Geometry check sheet. Reference: the model listing, model coordinates, mm. A direction names the side the tool comes from. Round coordinates to 2 decimals unless told otherwise and drop trailing zeros. Write each loop counter-clockwise with the first axis right and the second up, starting at its lowest first coordinate (ties: lowest second). Pieces come first, ordered by that corner, then holes.
Item 1: Cross-section at B-B (z = 44). Enter the section's corners in (x, y) (3 decimals), then the cut area to 3 significant figures.
Item 2: Cross-section at D-D (x = -25.5). Enter the section's corners in (y, z) (3 decimals).
Item 3: Access from +Z, -Z, +X, -X, +Y, -Y to the whole of each face (thin tool, end or side, straight path). Record for faces 1 (the face through (39.792, 7, 25)), 2 (the face through (66.286, -27.049, 10.43)), 3 (the face through (6, -10.997, 42)), 4 (the face through (-45.794, -30, 23)), 5 (the face through (-26.883, 7, 25)).
Item 4: Scan lines: probe 1 along X at (y, z) = (-36, 23); probe 2 along X at (y, z) = (-37, 5.5); probe 3 along Z at (x, y) = (-30.5, 4) (3 decimals). Record each from-to range of solid material in increasing order.
Item 5: Draft check along X on faces 6 (the face through (-54.41, -11.95, 30.41)), 7 (the face through (4, -20.522, 23)), 8 (the face through (4, -8, 0)). Enter one of: pulls with the +X half, pulls with the -X half, needs draft (parallel to the pull), parting line crosses it, or undercut.
Item 6: Cross-section at A-A (y = -22). Enter the section's corners in (x, z) (3 decimals).
Item 7: Cross-section at C-C (y = -5). Enter the section's corners in (x, z) (3 decimals).
Item 8: Depth check by flat-ended pin: P1, Ø20.5, axis at y = -24.5, z = 33.5, coming from the -X side; P2, Ø2, axis at x = 14, z = 34, coming from the -Y side; P3, Ø16.5, axis at x = 7, y = 6.5, coming from the +Z side; P4, Ø8.5, axis at x = 62.16, y = 9.35, coming from the -Z side. Enter the tip coordinate at first touch or a pass-through.
from build123d import *

# Parameters (mm, degrees)
SKETCH1_R             = 7.14375
BOSS_EXTRUDE1_DEPTH   = 9.525
BOSS_EXTRUDE1_2_DEPTH = 9.525
BOSS_EXTRUDE2_DEPTH   = 47.625
BOSS_EXTRUDE3_DEPTH   = 38.1
FILLET1_R             = 3.175


with BuildPart() as part:
    # Sketch1 → Boss-Extrude1 (new body)
    with BuildSketch(Plane.XY):
        Polygon((-26.883211679, -10.996624088), (-26.883211679, 22.340875912), (-71.194160584, 22.340875912), (-71.194160584, -39.571624088), (-55.319160584, -39.571624088), (-55.319160584, -10.996624088), align=None)
        with Locations(Location((-52.144160584, 8.053375912, 0), (0, 0, 180))):
            Circle(SKETCH1_R, mode=Mode.SUBTRACT)
    extrude(amount=BOSS_EXTRUDE1_DEPTH)



with BuildPart() as body_2:
    # Sketch1 → Boss-Extrude1 2 (new body)
    with BuildSketch(Plane.XY):
        Polygon((39.791788321, 22.340875912), (39.791788321, -10.996624088), (65.330839416, -10.996624088), (65.330839416, -39.571624088), (81.205839416, -39.571624088), (81.205839416, 22.340875912), align=None)
        with Locations(Location((62.155839416, 9.351186131, 0), (0, 0, 180))):
            Circle(SKETCH1_R, mode=Mode.SUBTRACT)
    extrude(amount=BOSS_EXTRUDE1_2_DEPTH)


with BuildPart() as part_1:
    add(part.part)

    add(body_2.part)  # Boss-Extrude2 merges body 2
    # Sketch1_4 → Boss-Extrude2 (add)
    with BuildSketch(Plane.XY):
        Polygon((39.791788321, -10.996624088), (-26.883211679, -10.996624088), (-55.319160584, -10.996624088), (-55.319160584, -39.571624088), (-45.794160584, -39.571624088), (-45.794160584, -37.984124088), (-45.794160584, -20.521624088), (55.805839416, -20.521624088), (55.805839416, -37.984124088), (55.805839416, -39.571624088), (65.330839416, -39.571624088), (65.330839416, -10.996624088), align=None)
    extrude(amount=BOSS_EXTRUDE2_DEPTH)

    # Sketch1_5 → Boss-Extrude3 (add)
    with BuildSketch(Plane.XY):
        with BuildLine():
            Line((-17.219160584, 22.340875912), (-26.883211679, 22.340875912))
            Line((-26.883211679, 22.340875912), (-26.883211679, -10.996624088))
            Line((-26.883211679, -10.996624088), (39.791788321, -10.996624088))
            Line((39.791788321, -10.996624088), (39.791788321, 22.340875912))
            Line((39.791788321, 22.340875912), (27.230839416, 22.340875912))
            ThreePointArc((27.230839416, 22.340875912), (5.005839416, 0.115875912), (-17.219160584, 22.340875912))
        make_face()
    extrude(amount=BOSS_EXTRUDE3_DEPTH)

    # Fillet1
    fillet1_edges = [part_1.edges().sort_by_distance(p)[0] for p in [
        (-41.101186131, -10.996624088, 9.525),
        (-26.883211679, 5.672125912, 9.525),
        (65.330839416, -10.996624088, 28.575),
        (-55.319160584, -10.996624088, 28.575),
        (39.791788321, 5.672125912, 9.525),
        (52.561313869, -10.996624088, 9.525),
        (65.330839416, -25.284124088, 9.525),
        (-26.883211679, -10.996624088, 23.8125),
        (39.791788321, -10.996624088, 23.8125),
        (-55.319160584, -25.284124088, 9.525),
    ]]
    fillet(fillet1_edges, radius=FILLET1_R)


solid = part_1.part
Resolved:
1. outline: (-55.319, -39.572) - (-45.794, -39.572) - (-45.794, -20.522) - (55.806, -20.522) - (55.806, -39.572) - (65.331, -39.572) - (65.331, -14.172) arc R3.175 ccw to (62.156, -10.997) - (-52.144, -10.997) arc R3.175 ccw to (-55.319, -14.172) - close
1. area: 1,510 mm2
2. outline: (-20.522, 0) - (22.341, 0) - (22.341, 38.1) - (-10.997, 38.1) - (-10.997, 47.625) - (-20.522, 47.625) - close
3. face 1: +Z, +X, +Y
3. face 2: +Z, +X, +Y, -Y
3. face 3: +Z, +Y
3. face 4: +Z, -Z, -Y
3. face 5: +Z, -X, +Y
4. probe 1: x = -55.32 to -45.79, 55.81 to 65.33
4. probe 2: x = -71.19 to -45.79, 55.81 to 81.21
4. probe 3: z = 0 to 9.525
5. face 6: pulls with the -X half
5. face 7: undercut
5. face 8: needs draft
6. outline: (-71.194, 0) - (-45.794, 0) - (-45.794, 47.625) - (-55.319, 47.625) - (-55.319, 12.7) arc R3.175 cw to (-58.494, 9.525) - (-71.194, 9.525) - close; (55.806, 0) - (81.206, 0) - (81.206, 9.525) - (68.506, 9.525) arc R3.175 cw to (65.331, 12.7) - (65.331, 47.625) - (55.806, 47.625) - close
7. outline: (-71.194, 0) - (81.206, 0) - (81.206, 9.525) - (42.967, 9.525) arc R3.175 cw to (39.792, 12.7) - (39.792, 38.1) - (-26.883, 38.1) - (-26.883, 12.7) arc R3.175 cw to (-30.058, 9.525) - (-71.194, 9.525) - close
8. P1: stops at x = -55.32
8. P2: stops at y = -20.52
8. P3: stops at z = 38.1
8. P4: passes through
